Autodesk Fusion 360 part; units mm, degrees
sketch "スケッチ1" plane through (0, 0, 0) normal (0, 0, 1) x (1, 0, 0)
  line L0 (19.2851, -21.7594) -> (19.2851, -31.7595)
  line L1 (19.2851, -31.7595) -> (16.7852, -31.7595)
  line L2 (16.7852, -21.7594) -> (19.2851, -21.7594)
  line L3 (16.7852, -41.7596) -> (19.2851, -41.7596)
  line L4 (16.7852, -31.7595) -> (16.7852, -41.7596)
  line L5 (16.7852, -11.7593) -> (16.7852, -21.7594)
  line L6 (21.0353, -61.7598) -> (21.0353, -64.2597)
  line L7 (19.2851, -41.7596) -> (19.2851, -51.7597)
  line L8 (30.2852, -11.7593) -> (16.7852, -11.7593)
  line L9 (21.0353, -64.2597) -> (26.0353, -64.2597)
  line L10 (27.7852, -51.7597) -> (30.2852, -51.7597)
  line L11 (26.0353, -61.7598) -> (27.7852, -61.7598)
  line L12 (16.7852, -51.7597) -> (16.7852, -61.7598)
  line L13 (16.7852, -61.7598) -> (21.0353, -61.7598)
  line L14 (19.2851, -51.7597) -> (16.7852, -51.7597)
  line L15 (26.0353, -64.2597) -> (26.0353, -61.7598)
  line L16 (27.7852, -61.7598) -> (27.7852, -51.7597)
  line L17 (30.2852, -51.7597) -> (30.2852, -11.7593)
extrude "押し出し1" add sketch "スケッチ1" along normal blind 2.5
Geometry: final body of the model. Coordinates: model frame, mm. A direction names the side the tool comes from. Round coordinates to 2 decimals unless told otherwise and drop trailing zeros. Order: outer loops, then holes, each group sorted by start corner. A loop starts at its lowest first (then second) coordinate and runs counter-clockwise, first axis right, second up. Notation, with made-up numbers: (-29, -28.5) - (30, -28.5) arc R13 ccw to (30, -13.5) - close; hole circle Ø10 at (11, 16.5). An arc over 180 degrees is marked (long way). Write item = value, one per line. Start each with the question number.
Q1. Ray query, line 1 (Y direction, x = 21, z = 0.4); line 2 (X direction, y = -30.5, z = 1); line 3 (X direction, y = -53, z = 1.25). Return the intervals inside material, ascending. Write a range as from..to.
Q2. Pin query (flat end, axial travel): pin 1 (1.2 mm diameter, centred on x = 19, z = 1, fed in from -Y); pin 2 (0.7 mm diameter, centred on y = -63.5, z = 1, fed in from -X). Return the tip coordinate at first contact, or that it passes through.
Q3. Pull-direction query (Y, two-part tool) for faces 6 (the flat face through (29, -51.76, 1)), 7 (the flat face through (19.285, -27, 1)), 8 (the flat face through (23, -38, 2.5)); classes: +Y half, -Y half, draft (parallel to the pull), parting line (faces both ways), or undercut.
Q4. Cut plane B-B on y = -47.5. Return the cut outline in (x, z), and give its area (3 significant figures).
Q5. Cut plane C-C on x = 29.5. Return the cut outline in (y, z).
Q6. Access query for faces 1 (the flat face through (21.035, -63, 1)), 2 (the flat face through (16.785, -37, 1)), 3 (the flat face through (18, -31.76, 1)), 4 (the flat face through (27.785, -57, 1)), 5 (the flat face through (30.285, -32, 1)). Directions: +Z, -Z, +X, -X, +Y, -Y. A direction counts if a zero-diameter tool reaches every point of the face in a straight line with its end or side. Return the directions, or none.
Q7. Cut plane A-A on z = 0.7. Return the cut outline in (x, y).
Outcome:
q1.line_1 = -61.76..-11.76
q1.line_2 = 19.29..30.29
q1.line_3 = 16.79..27.79
q2.pin_1 = -61.76
q2.pin_2 = 21.04
q3.face_6 = -Y half
q3.face_7 = undercut
q3.face_8 = draft
q4.outline = (19.29, 0) - (30.29, 0) - (30.29, 2.5) - (19.29, 2.5) - close
q4.area = 27.5 mm^2
q5.outline = (-51.76, 0) - (-11.76, 0) - (-11.76, 2.5) - (-51.76, 2.5) - close
q6.face_1 = +Z, -Z, -X, -Y
q6.face_2 = +Z, -Z, -X, +Y, -Y
q6.face_3 = +Z, -Z, -X
q6.face_4 = +Z, -Z, +X, -Y
q6.face_5 = +Z, -Z, +X, +Y, -Y
q7.outline = (16.79, -61.76) - (21.04, -61.76) - (21.04, -64.26) - (26.04, -64.26) - (26.04, -61.76) - (27.79, -61.76) - (27.79, -51.76) - (30.29, -51.76) - (30.29, -11.76) - (16.79, -11.76) - (16.79, -21.76) - (19.29, -21.76) - (19.29, -31.76) - (16.79, -31.76) - (16.79, -41.76) - (19.29, -41.76) - (19.29, -51.76) - (16.79, -51.76) - close
